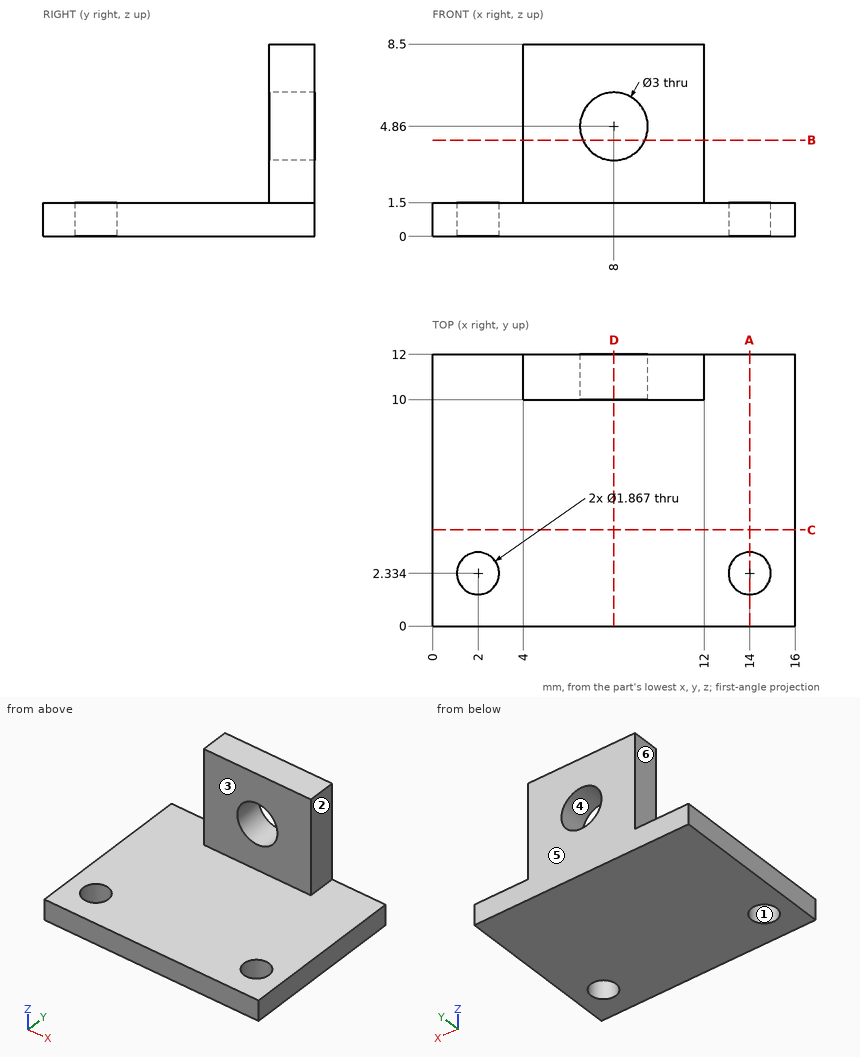
Geometry check sheet. Reference: drawing and pictorial views, mm from the part's lowest x, y, z. A direction names the side the tool comes from. Give positions to 0.01 mm unless a question says otherwise; leave off trailing zeros. Order: outer loops, then holes, each group sorted by start corner. A loop starts at its lowest first (then second) coordinate and runs counter-clockwise, first axis right, second up. Notation, with made-up numbers: M 34,46 L 92,46 A14 ccw 92,55 Z; hole C 45.5,-7 d11. An arc over 180 degrees is marked long. Answer in a Markdown table with one row per item.
1) Cross-section at C-C, the plane y = 4.25. Enter the section's corners in (x, z).
Filled sheet:
| item | result |
|---|---|
| outline | M 0,0 L 16,0 L 16,1.5 L 0,1.5 Z |
2) Cross-section at B-B, the plane z = 4.25. Enter the section's corners in (x, y), plus the area to 3 significant figures.
Filled sheet:
| item | result |
|---|---|
| outline | M 4,10 L 6.63,10 L 6.63,12 L 4,12 Z; M 9.37,10 L 12,10 L 12,12 L 9.37,12 Z |
| area | 10.5 mm2 |
3) Cross-section at A-A, the plane x = 14. Enter the section's corners in (y, z).
Filled sheet:
| item | result |
|---|---|
| outline | M 0,0 L 1.4,0 L 1.4,1.5 L 0,1.5 Z; M 3.27,0 L 12,0 L 12,1.5 L 3.27,1.5 Z |
4) Gauge pin test, flat ends, axial feed: P1, Ø1.5, axis at x = 14, y = 2.33, coming from the +Z side; P2, Ø1.6, axis at y = 10.5, z = 3.5, coming from the -X side; P3, Ø1, axis at y = 11, z = 5.5, coming from the +X side. Record the tip position at first contact, or that the pin passes through.
Filled sheet:
| item | result |
|---|---|
| P1 | passes through |
| P2 | stops at x = 4 |
| P3 | stops at x = 12 |
5) Cross-section at D-D, the plane x = 8. Enter the section's corners in (y, z).
Filled sheet:
| item | result |
|---|---|
| outline | M 0,0 L 12,0 L 12,3.36 L 10,3.36 L 10,1.5 L 0,1.5 Z; M 10,6.36 L 12,6.36 L 12,8.5 L 10,8.5 Z |
6) Access from +Z, -Z, +X, -X, +Y, -Y to the whole of each face (thin tool, end or side, straight path). Record for the marked faces 5 and 6.
Filled sheet:
| item | result |
|---|---|
| face 5 | +Z, -Z, +X, -X, +Y |
| face 6 | +Z, -X, +Y, -Y |
7) Thickness scan on L1, parallel to Z at x = 8, y = 11.3; L2, parallel to Z at x = 4.75, y = 7; L3, parallel to Y at x = 2, z = 1.25. Record the ranges inside material, lowest first. Write a range as [from, to].
Filled sheet:
| item | result |
|---|---|
| L1 | z = [0, 3.36], [6.36, 8.5] |
| L2 | z = [0, 1.5] |
| L3 | y = [0, 1.4], [3.27, 12] |
8) Release check for a two-part mould opening along X. For the marked faces 1, 2, 3 and 4 record: +X half, -X half, draft (parallel to the pull), parting line (faces both ways), or undercut.
Filled sheet:
| item | result |
|---|---|
| face 1 | undercut |
| face 2 | +X half |
| face 3 | draft |
| face 4 | undercut |
